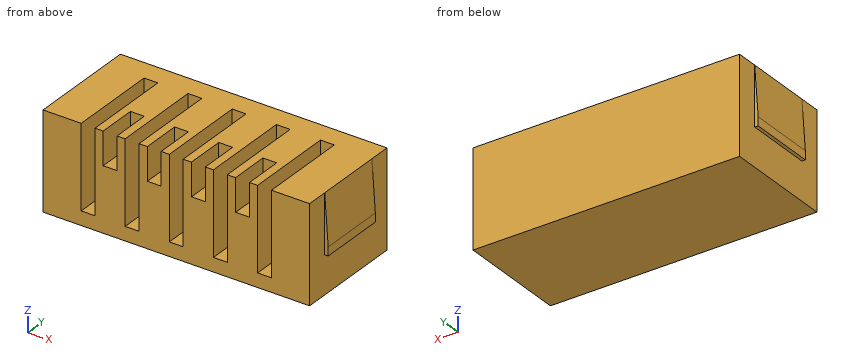
```python
from build123d import *

# Parameters (mm, degrees)
SKETCH1_W           = 15.4
SKETCH1_H           = 6.4
BOSS_EXTRUDE1_DEPTH = 5.6
SKETCH2_W           = 0.8
SKETCH2_H           = 4.8
SKETCH2_H_2         = 1.9
CUT_EXTRUDE1_DEPTH  = 5.2
SKETCH3_W           = 3.4
SKETCH3_H           = 3.9
BOSS_EXTRUDE2_DEPTH = 0.2
CUT_EXTRUDE2_REACH  = 12.968
SKETCH5_W           = 0.8
SKETCH5_H           = 2.945
BOSS_EXTRUDE3_DEPTH = 1.9


with BuildPart() as part:
    # Sketch1 → Boss-Extrude1 (new body)
    with BuildSketch(Plane.XY):
        Rectangle(SKETCH1_W, SKETCH1_H)
    extrude(amount=BOSS_EXTRUDE1_DEPTH)

    # Sketch2 → Cut-Extrude1 (cut)
    with BuildSketch(Plane.XZ.offset(3.2)):
        with Locations((5.095, 3.2)):
            Rectangle(SKETCH2_W, SKETCH2_H)
        with Locations((2.545, 3.2)):
            Rectangle(SKETCH2_W, SKETCH2_H)
        with Locations((-0.005, 3.2)):
            Rectangle(SKETCH2_W, SKETCH2_H)
        with Locations((-2.555, 3.2)):
            Rectangle(SKETCH2_W, SKETCH2_H)
        with Locations((-5.095, 3.2)):
            Rectangle(SKETCH2_W, SKETCH2_H)
        with Locations((3.825, 4.65)):
            Rectangle(SKETCH2_W, SKETCH2_H_2)
        with Locations((1.275, 4.65)):
            Rectangle(SKETCH2_W, SKETCH2_H_2)
        with Locations((-1.275, 4.65)):
            Rectangle(SKETCH2_W, SKETCH2_H_2)
        with Locations((-3.825, 4.65)):
            Rectangle(SKETCH2_W, SKETCH2_H_2)
    extrude(amount=-CUT_EXTRUDE1_DEPTH, mode=Mode.SUBTRACT)

    # Sketch3 → Boss-Extrude2 (add)
    with BuildSketch(Plane(origin=(7.7, 0, 0), x_dir=(0, 0, -1), z_dir=(1, 0, 0))):
        with Locations((-3.9, 0)):
            Rectangle(SKETCH3_W, SKETCH3_H)
    boss_extrude2 = extrude(amount=BOSS_EXTRUDE2_DEPTH)

    # Sketch4 → Cut-Extrude2 (cut, up to next)
    with BuildSketch(Plane(origin=(0, 1.95, 0), x_dir=(1, 0, 0), z_dir=(0, 1, 0)), mode=Mode.PRIVATE) as cut_extrude2_sk1:
        Polygon((7.9, -2.7), (7.7, -5.6), (7.9, -5.6), align=None)
    cut_extrude2_tool1 = extrude(cut_extrude2_sk1.sketch, amount=-CUT_EXTRUDE2_REACH, mode=Mode.PRIVATE) & part.part
    cut_extrude2 = cut_extrude2_tool1.solids().sort_by_distance((7.833333, 1.95, 4.633333))[0]
    add(cut_extrude2, mode=Mode.SUBTRACT)

    # Mirror1: Boss-Extrude2, Cut-Extrude2 across plane
    add(boss_extrude2.mirror(Plane(origin=(0, 0, 0), x_dir=(0, 0, 1), z_dir=(1, 0, 0))))
    add(cut_extrude2.mirror(Plane(origin=(0, 0, 0), x_dir=(0, 0, 1), z_dir=(1, 0, 0))), mode=Mode.SUBTRACT)

    # Sketch5 → Boss-Extrude3 (add)
    with BuildSketch(Plane.XY.offset(3.7)):
        with Locations((-3.825, 0.5275)):
            Rectangle(SKETCH5_W, SKETCH5_H)
        with Locations((-1.275, 0.5275)):
            Rectangle(SKETCH5_W, SKETCH5_H)
        with Locations((1.275, 0.5275)):
            Rectangle(SKETCH5_W, SKETCH5_H)
        with Locations((3.825, 0.5275)):
            Rectangle(SKETCH5_W, SKETCH5_H)
    extrude(amount=BOSS_EXTRUDE3_DEPTH)


solid = part.part
```
The listing builds one solid part. Answer for the finished solid, in the listing's coordinates (mm). Give positions to 0.01 mm unless a question says otherwise; leave off trailing zeros. Write each loop counter-clockwise with the first axis right and the second up, starting at its lowest first coordinate (ties: lowest second). Pieces come first, ordered by that corner, then holes. Notation, with made-up numbers: (57, 56.25) -> (74, 56.25) arc R12 ccw to (74, 79.25) -> close; hole circle Ø9 at (-13.5, 5). An arc over 180 degrees is marked (long way). Write item = value, one per line. Start each with the question number.
1) The part is cut by section C-C, the plane x = -2.5. Determine the outline of the cut face in (y, z), and give its area (3 significant figures).
2) Straight lines are drawn through the part: line 1 along X through (y, z) = (1, 1.7) (3 decimals); line 2 along X through (y, z) = (-1.5, 3.25) (3 decimals); line 3 along Y through (x, z) = (0, 3.1). For each, find the intervals that lie inside material, in ascending order.
3) Each of these flat-tipped pins is pushed along its axis until it touches: pin 1 (1 mm diameter, centred on y = -1, z = 4.5, fed in from -X); pin 2 (2.5 mm diameter, centred on y = -1.5, z = 4, fed in from -X); pin 3 (1.5 mm diameter, centred on y = -2, z = 5, fed in from +X). Where does it stop, or does it pass through?
4) The part is cut by section D-D, the plane z = 0.45. Determine the outline of the cut face in (x, y), and give its area (3 significant figures).
Solutions:
q1.outline = (-3.2, 0) -> (3.2, 0) -> (3.2, 5.6) -> (2, 5.6) -> (2, 0.8) -> (-3.2, 0.8) -> close
q1.area = 10.9 mm²
q2.line_1 = -7.7 to -5.495, -4.695 to -2.955, -2.155 to -0.405, 0.395 to 2.145, 2.945 to 4.695, 5.495 to 7.7
q2.line_2 = -7.862 to -5.495, -4.695 to -2.955, -2.155 to -0.405, 0.395 to 2.145, 2.945 to 4.695, 5.495 to 7.862
q2.line_3 = 2 to 3.2
q3.pin_1 = -7.81
q3.pin_2 = -7.9
q3.pin_3 = 7.79
q4.outline = (-7.7, -3.2) -> (7.7, -3.2) -> (7.7, 3.2) -> (-7.7, 3.2) -> close
q4.area = 98.6 mm²
